Geometry: see drawing. Coordinates: mm, zero at the bounding-box minimum. A direction names the side the tool comes from. Coordinates: 2 decimals unless noted, no trailing zeros. Loops run counter-clockwise (first coordinate to the right, second up) from the corner with the lowest first, then second, coordinate; pieces in that order, holes last. Notation, with made-up numbers: (-29.5, 53.5) -> (-11.5, 53.5) arc R34 cw to (-11.5, 84.5) -> close; hole circle Ø10 at (4.25, 55.25). An arc over 180 degrees is marked (long way). One line per item, written item: value. Start each with the question number.
Item 1: Section query B-B on z = 16. Return loops of the section in (x, y) (1 decimal), then the cut area to 3 significant figures.
Item 2: Set-up query: the marked faces 1 and 2. Return all of +Z, -Z, +X, -X, +Y, -Y with unobstructed straight access to the full face (end or side cutting, diameter ignored); none if empty.
Item 3: Section query A-A on y = 69.85. Return loops of the section in (x, z) (1 decimal), then the cut area to 3 significant figures.
Item 4: Section query C-C on x = 65.5. Return loops of the section in (y, z) (1 decimal).
Item 5: Contact query for flat-ended pins moving along their axis: pin 1 Ø6 at (x, y) = (55.5, 127.5) entering from +Z (1 decimal); pin 2 Ø3.5 at (x, z) = (1, 33.5) entering from +Y; pin 3 Ø3.5 at (x, z) = (2, 48.5) entering from -Y; pin 4 Ø1.5 at (y, z) = (49, 25.5) entering from -X. Output: stop coordinate, or through.
Item 6: Ray query, probe 1 along X at (y, z) = (80, 60) (1 decimal); probe 2 along Z at (x, y) = (1, 69) (1 decimal). Return the intervals inside material, ascending. Write a range as from..to.
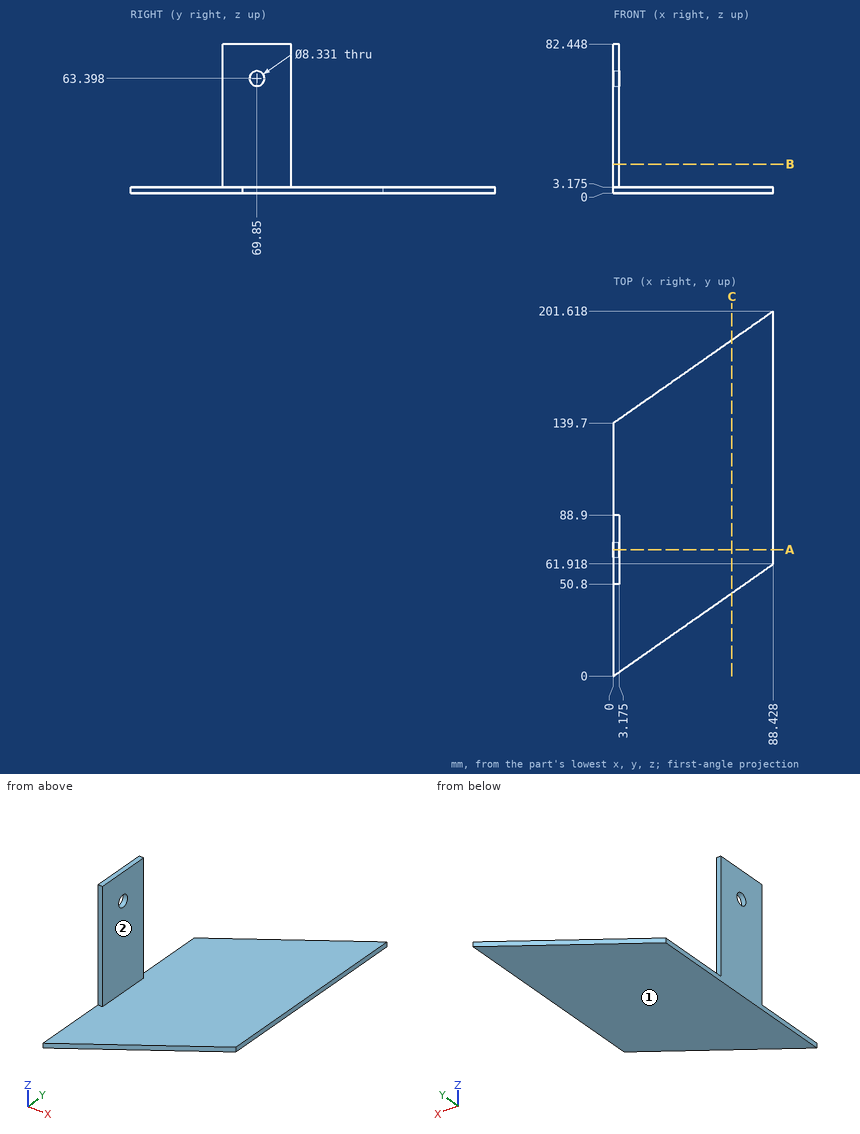
Reply:
1. outline: (0, 50.8) -> (3.2, 50.8) -> (3.2, 88.9) -> (0, 88.9) -> close
1. area: 121 mm²
2. face 1: -Z, +X, -X, +Y, -Y
2. face 2: +Z, +X, +Y, -Y
3. outline: (0, 0) -> (88.4, 0) -> (88.4, 3.2) -> (3.2, 3.2) -> (3.2, 59.2) -> (0, 59.2) -> close; (0, 67.6) -> (3.2, 67.6) -> (3.2, 82.4) -> (0, 82.4) -> close
3. area: 506 mm²
4. outline: (45.9, 0) -> (185.6, 0) -> (185.6, 3.2) -> (45.9, 3.2) -> close
5. pin 1: stops at z = 3.2
5. pin 2: stops at y = 88.9
5. pin 3: stops at y = 50.8
5. pin 4: passes through
6. probe 1: x = 0..3.2
6. probe 2: z = 0..59.3, 67.5..82.4
